Autodesk Inventor part; units mm, degrees
ref_plane "YZ Plane" through (0, 0, 0) normal (1, 0, 0) x (0, 1, 0)
ref_plane "XZ Plane" through (0, 0, 0) normal (0, 1, 0) x (-1, 0, 0)
ref_plane "XY Plane" through (0, 0, 0) normal (0, 0, 1) x (1, 0, 0)
sketch "Boceto1" plane through (0, 0, 0) normal (0, 0, 1) x (1, 0, 0)
  line L0 (8.9, -10) -> (-8.9, -10)
  line L1 (-8.9, -10) -> (-8.9, 10)
  line L2 (-8.9, 10) -> (8.9, 10)
  line L3 (8.9, 10) -> (8.9, -10)
  line L4 (8.9, -10) -> (-8.9, 10) construction
  line L5 (-8.9, -10) -> (8.9, 10) construction
  line L6 (0, 10) -> (0, -10)
  line L7 (8.9, 0) -> (-8.9, 0)
  line L8 (0, -3) -> (0, 3) construction
  line L9 (3, -3) -> (3, 3)
  line L10 (-3, 3) -> (-3, -3)
  arc A0 (-3, -3) -> (3, -3) centre (0, -3) ccw
  arc A1 (3, 3) -> (-3, 3) centre (0, 3) ccw
  point P0 (0, 0)
  dimension "d0" = 17.8
  dimension "d1" = 20
  dimension "d2" = 6
  dimension "d3" = 6
extrude "Extrusión1" add sketch "Boceto1" along normal blind 3 contours L0 L6 A0 L9 L7 L3 | L0 L1 L7 L10 A0 L6 | L7 L9 A1 L6 L2 L3 | L1 L2 L6 A1 L10 L7
sketch "Boceto2" plane through (0, 0, 3) normal (0, 0, 1) x (1, 0, 0)
  line L0 (-8.9, 10) -> (-8.9, -10)
  line L1 (-8.9, -10) -> (8.9, -10)
  line L2 (-8.9, -7) -> (8.9, -7)
  line L3 (8.9, -7) -> (8.9, -10)
  line L4 (8.9, -10) -> (-8.9, -10)
  line L5 (-8.9, -10) -> (-8.9, -7)
  point P0 (0, 0)
  dimension "d6" = 3
extrude "Extrusión2" add sketch "Boceto2" along normal blind 20
sketch "Boceto3" plane through (8.9, -10, 0) normal (1, 0, 0) x (0, 0, -1)
  line L0 (-3, 20) -> (-3, 3)
  line L1 (-3, 3) -> (-23, 3)
  line L2 (-3, 20) -> (-23, 3)
  line L3 (-23, 3) -> (-3, 3)
  line L4 (-3, 3) -> (-3, 20)
  point P0 (0, 10)
extrude "Extrusión3" add sketch "Boceto3" against normal blind 2.25
sketch "Boceto4" plane through (-8.9, -10, 0) normal (-1, 0, 0) x (0, 0, 1)
  line L0 (3, 20) -> (23, 3)
  line L1 (3, 20) -> (23, 3)
  line L2 (3, 3) -> (23, 3)
  line L3 (23, 3) -> (3, 3)
  line L4 (3, 3) -> (3, 20)
  point P0 (0, 10)
extrude "Extrusión4" add sketch "Boceto4" against normal blind 2.25
sketch "Boceto5" plane through (6.65, -7, 23) normal (0, 1, 0) x (1, 0, 0)
  line L0 (-6.65, 23) -> (-6.65, 0)
  line L1 (-15.55, 0) -> (2.25, 0)
  line L2 (2.25, 20) -> (2.25, 0)
  line L3 (-15.55, 23) -> (-15.55, 0)
  line L4 (2.25, 11.5) -> (-15.55, 11.5)
  line L5 (2.25, 23) -> (-15.55, 23)
  line L6 (-6.65, 14.5) -> (-6.65, 8.5) construction
  line L7 (-9.65, 14.5) -> (-9.65, 8.5)
  line L8 (-3.65, 8.5) -> (-3.65, 14.5)
  arc A0 (-3.65, 14.5) -> (-9.65, 14.5) centre (-6.65, 14.5) ccw
  arc A1 (-9.65, 8.5) -> (-3.65, 8.5) centre (-6.65, 8.5) ccw
  point P0 (-6.65, 11.5)
  dimension "d13" = 23
  dimension "d14" = 11.5
  dimension "d15" = 6
  dimension "d16" = 6
extrude "Extrusión5" cut sketch "Boceto5" against normal through all contours A0 L8 L4 L0 | L0 L4 L7 A0 | L4 L8 A1 L0 | L0 A1 L7 L4
properties part number "Cast corner bracket-20x20x17" material "Aluminio 6061, soldado"
Could you check a few things on this model? Use its own coordinates, in mm. A direction names the side the tool comes from. Give positions to 0.01 mm unless a question says otherwise; leave off trailing zeros. Order: outer loops, then holes, each group sorted by start corner. A loop starts at its lowest first (then second) coordinate and runs counter-clockwise, first axis right, second up.
Item 1: If we section it at C-C, the plane y = -1.25: Write out the boundary of the cut face in (x, z), plus the area to 3 significant figures.
Item 2: If we section it at A-A, the plane x = 0: Write out the boundary of the cut face in (y, z).
Item 3: If we mould it in two halves opening along Z, with no side actions, what happens to faces 5 (the face through (-3, 4, 3)), 6 (the face through (-3, -8, 11)), 7 (the face through (8.9, -2, 9))? For each: pulls with the +Z half, pulls with the -Z half, needs draft (parallel to the pull), parting line crosses it, or undercut.
Item 4: For faces 1 (the face through (-0.1, -8.5, 17.5)), 2 (the face through (6.65, -2, 9)), 3 (the face through (0, -6, 1)), 4 (the face through (4, 0, 0)), which set-ups out of +Z, -Z, +X, -X, +Y, -Y let a thin tool reach every point of the face, with its end or its side?
Item 5: If we section it at B-B, the plane z = 7.25: Write out the boundary of the cut face in (x, y), plus the area to 3 significant figures.
Item 6: I need wall thicknesses on line 1 (X direction, y = -5.25, z = 14.5); line 2 (X direction, y = -9, z = 10.5); line 3 (Y direction, x = -6.5, z = 10.5). Which ranges of each line are inside material? Lowest first, please.
Item 7: I'm going to push flat-ended pins straight in: pin 1 (1.5 mm diameter, centred on x = -4, y = 7.5, fed in from +Z); pin 2 (4 mm diameter, centred on x = 1.5, z = 12, fed in from +Y). Where does each tip first touch, or does it pass through?
Item 8: If we section it at D-D, the plane x = 4: Write out the boundary of the cut face in (y, z), plus the area to 3 significant figures.
Values:
1. outline: (-8.9, 0) - (-3, 0) - (-3, 3) - (-6.65, 3) - (-6.65, 16.24) - (-8.9, 16.24) - close; (3, 0) - (8.9, 0) - (8.9, 16.24) - (6.65, 16.24) - (6.65, 3) - (3, 3) - close
1. area: 95.0 mm2
2. outline: (-10, 0) - (-6, 0) - (-6, 3) - (-7, 3) - (-7, 5.5) - (-10, 5.5) - close; (-10, 17.5) - (-7, 17.5) - (-7, 23) - (-10, 23) - close; (6, 0) - (10, 0) - (10, 3) - (6, 3) - close
3. face 5: pulls with the +Z half
3. face 6: undercut
3. face 7: needs draft
4. face 1: +Y, -Y
4. face 2: +Z, +Y
4. face 3: +Z, -Z
4. face 4: -Z, +X, -X, +Y, -Y
5. outline: (-8.9, -10) - (-2.73, -10) - (-2.73, -7) - (-6.65, -7) - (-6.65, 6.39) - (-8.9, 6.39) - close; (2.73, -10) - (8.9, -10) - (8.9, 6.39) - (6.65, 6.39) - (6.65, -7) - (2.73, -7) - close
5. area: 97.3 mm2
6. line 1: x = -8.9 to -6.65, 6.65 to 8.9
6. line 2: x = -8.9 to -3, 3 to 8.9
6. line 3: y = -10 to -7
7. pin 1: stops at z = 3
7. pin 2: stops at y = -7
8. outline: (-10, 0) - (10, 0) - (10, 3) - (-7, 3) - (-7, 23) - (-10, 23) - close
8. area: 120 mm2
